Geometry: final body of the model. Coordinates: model frame, mm. A direction names the side the tool comes from. Give positions to 0.01 mm unless a question says otherwise; leave off trailing zeros. Order: outer loops, then holes, each group sorted by start corner. A loop starts at its lowest first (then second) coordinate and runs counter-clockwise, first axis right, second up. Notation, with made-up numbers: (-5, 43.5) - (20, 43.5) arc R22 cw to (20, 66.5) - close; hole circle Ø8 at (29, 73.5). An arc over 180 degrees is marked (long way). Write item = value, one per line. Start each with the question number.
from build123d import *

# Parameters (mm, degrees)
SKETCH1_R           = 80
BOSS_EXTRUDE1_DEPTH = 4
SKETCH2_R           = 65
SKETCH2_R_2         = 60
BOSS_EXTRUDE2_DEPTH = 3
SKETCH3_R           = 3
CUT_EXTRUDE2_DEPTH  = 8
SKETCH5_R           = 27.5
CUT_EXTRUDE4_DEPTH  = 8


with BuildPart() as part:
    # Sketch1 → Boss-Extrude1 (new body)
    with BuildSketch(Plane.XY):
        Circle(SKETCH1_R)
    extrude(amount=BOSS_EXTRUDE1_DEPTH)

    # Sketch2 → Boss-Extrude2 (add)
    with BuildSketch(Plane.XY.offset(4)):
        Circle(SKETCH2_R)
        Circle(SKETCH2_R_2, mode=Mode.SUBTRACT)
    extrude(amount=BOSS_EXTRUDE2_DEPTH)

    # Sketch3 → Cut-Extrude2 (cut, through all)
    with BuildSketch(Plane(origin=(0, 0, 0), x_dir=(-1, 0, 0), z_dir=(0, 0, -1))):
        with Locations((0, 70)):
            Circle(SKETCH3_R)
        with Locations((60.621778265, -35)):
            Circle(SKETCH3_R)
        with Locations((-60.621778265, -35)):
            Circle(SKETCH3_R)
    extrude(amount=-CUT_EXTRUDE2_DEPTH, mode=Mode.SUBTRACT)

    # Sketch5 → Cut-Extrude4 (cut, through all)
    with BuildSketch(Plane.XY):
        Circle(SKETCH5_R)
    extrude(amount=CUT_EXTRUDE4_DEPTH, mode=Mode.SUBTRACT)


solid = part.part
Q1. Section D-D, the plane x = 25. Return the cut outline in (y, z), then the cut area to 3 significant figures.
Q2. Pull-direction query (X, two-part tool) for faces 1 (the cylindrical face through (-5.961, -26.846, 1.972)), 2 (the flat face through (-6, 66, 4)), 3 (the cylindrical face through (-17.34, -78.1, 1.97)); classes: +X half, -X half, draft (parallel to the pull), parting line (faces both ways), or undercut.
Q3. Material intervals for line 1 along Y through (x, z) = (0, 0.8); line 2 along Y through (x, z) = (0, 5.8); line 3 along Z through (x, y) = (72.5, -21.5), sorted ascending. Write a range as from..to.
Q4. Contact query for flat-ended pins moving along their axis: pin 1 (3.5 mm diameter, centred on x = -60.62, y = -35, fed in from +Z); pin 2 (5 mm diameter, centred on x = -38, y = 34, fed in from +Z); pin 3 (2 mm diameter, centred on y = 62.5, z = 1, fed in from +X); pin 4 (2 mm diameter, centred on x = -6.5, z = 2.5, fed in from +Y). Output: stop coordinate, or through.
Q5. Section A-A, the plane y = 0. Return the cut outline in (x, z), then the cut area to 3 significant figures.
Q6. Set-up query: faces 4 (the flat face through (-1, -34, 0)), 5 (the cylindrical face through (-59.94, 2.64, 5.48)). Return all of +Z, -Z, +X, -X, +Y, -Y with unobstructed straight access to the full face (end or side cutting, diameter ignored); none if empty.
Q7. Section C-C, the plane z = 2.5. Return the cut outline in (x, y).
Q8. Section B-B, the plane x = 0. Return the cut outline in (y, z), then the cut area to 3 significant figures.
The answers:
q1.outline = (-75.99, 0) - (-11.46, 0) - (-11.46, 4) - (-54.54, 4) - (-54.54, 7) - (-60, 7) - (-60, 4) - (-75.99, 4) - close; (11.46, 0) - (75.99, 0) - (75.99, 4) - (60, 4) - (60, 7) - (54.54, 7) - (54.54, 4) - (11.46, 4) - close
q1.area = 549 mm²
q2.face_1 = undercut
q2.face_2 = draft
q2.face_3 = parting line
q3.line_1 = -80..-27.5, 27.5..67, 73..80
q3.line_2 = -65..-60, 60..65
q3.line_3 = 0..4
q4.pin_1 = through
q4.pin_2 = 4
q4.pin_3 = 51.16
q4.pin_4 = 79.81
q5.outline = (-80, 0) - (-27.5, 0) - (-27.5, 4) - (-60, 4) - (-60, 7) - (-65, 7) - (-65, 4) - (-80, 4) - close; (27.5, 0) - (80, 0) - (80, 4) - (65, 4) - (65, 7) - (60, 7) - (60, 4) - (27.5, 4) - close
q5.area = 450 mm²
q6.face_4 = -Z, +X, -X, +Y, -Y
q6.face_5 = +Z
q7.outline = circle Ø160 at (0, 0); hole circle Ø6 at (-60.62, -35); hole circle Ø55 at (0, 0); hole circle Ø6 at (0, 70); hole circle Ø6 at (60.62, -35)
q8.outline = (-80, 0) - (-27.5, 0) - (-27.5, 4) - (-60, 4) - (-60, 7) - (-65, 7) - (-65, 4) - (-80, 4) - close; (27.5, 0) - (67, 0) - (67, 4) - (65, 4) - (65, 7) - (60, 7) - (60, 4) - (27.5, 4) - close; (73, 0) - (80, 0) - (80, 4) - (73, 4) - close
q8.area = 426 mm²
